Job drawing, mm, ordinate dimensions from the low corner. One solid piece. A direction names the side the tool comes from. Coordinates: 2 decimals unless noted, no trailing zeros. Order: outer loops, then holes, each group sorted by start corner. A loop starts at its lowest first (then second) coordinate and runs counter-clockwise, first axis right, second up. Notation, with made-up numbers: (-16, 53) - (28, 53) arc R19 ccw to (28, 67) - close; hole circle Ø2 at (-9.5, 74.5). An arc over 180 degrees is marked (long way). Use a Markdown table: item, result. Add a question column.
1) Tool access for the marked faces 1 and 2: list every direction of +Z, -Z, +X, -X, +Y, -Y with a clear straight run to the whole face (end or side of a thin tool).
2) Two-plate mould, pull along X, no slides. Class the marked faces 3, 4 and 5: +X half, -X half, draft (parallel to the pull), parting line (faces both ways), or undercut.
3) Saw through at D-D on y = 45. List the corners of the cut face in (x, z).
4) Saw through at A-A on y = 27.5. List the corners of the cut face in (x, z).
5) Wall check: L1, parallel to X at y = 27, z = 7 (1 decimal); L2, parallel to Y at x = 28, z = 7 (1 decimal); L3, parallel to X at y = 46, z = 4.5 (1 decimal). Give the ranges that are in metal, low to high. Write a range as [from, to].
6) Saw through at B-B on x = 27.5. List the corners of the cut face in (y, z).
7) Saw through at C-C on z = 5.75. List the corners of the cut face in (x, y).
8) Drop flat-ended pins along their axis: P1, Ø3, axis at y = 38, z = 4.5, coming from the +X side; P2, Ø4, axis at x = 13.52, y = 10.84, coming from the +Z side; P3, Ø4, axis at x = 36.5, z = 6.5, coming from the +Y side; P4, Ø4, axis at x = 12.5, z = 2, coming from the -Y side. Give the stop position or say it passes through.
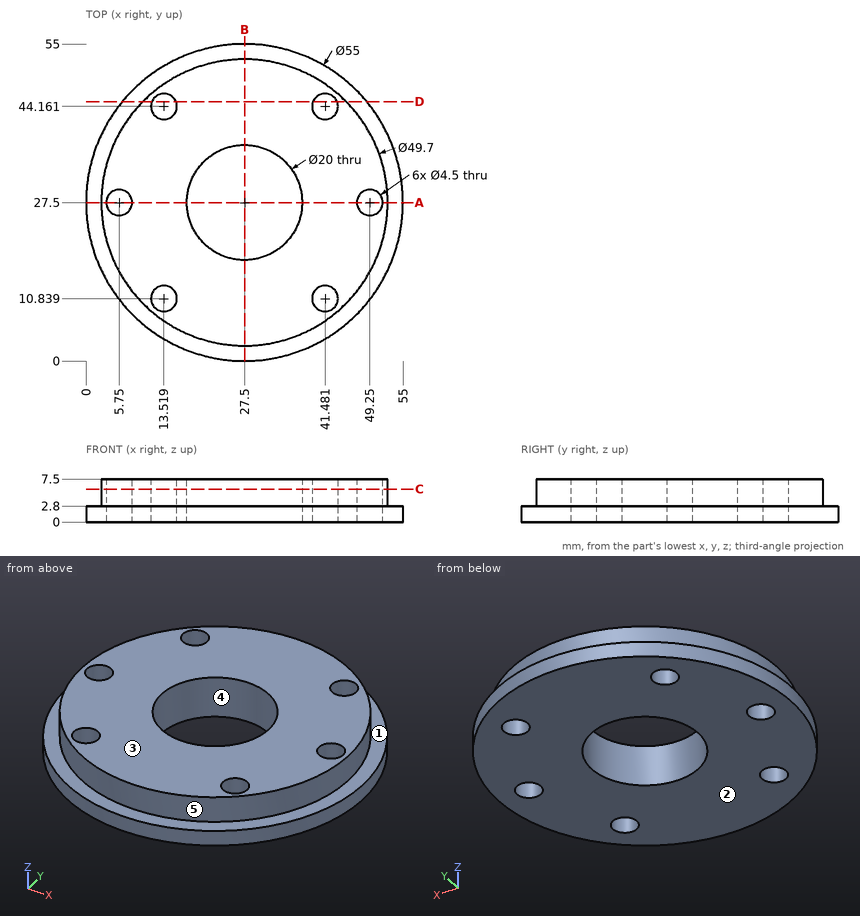
Results are:
| question | item | result |
|---|---|---|
| 1 | face 1 | +Z |
| 1 | face 2 | -Z, +X, -X, +Y, -Y |
| 2 | face 3 | draft |
| 2 | face 4 | undercut |
| 2 | face 5 | parting line |
| 3 | outline | (6.29, 0) - (11.43, 0) - (11.43, 7.5) - (9.86, 7.5) - (9.86, 2.8) - (6.29, 2.8) - close; (15.61, 0) - (39.39, 0) - (39.39, 7.5) - (15.61, 7.5) - close; (43.57, 0) - (48.71, 0) - (48.71, 2.8) - (45.14, 2.8) - (45.14, 7.5) - (43.57, 7.5) - close |
| 4 | outline | (0, 0) - (3.5, 0) - (3.5, 7.5) - (2.65, 7.5) - (2.65, 2.8) - (0, 2.8) - close; (8, 0) - (17.5, 0) - (17.5, 7.5) - (8, 7.5) - close; (37.5, 0) - (47, 0) - (47, 7.5) - (37.5, 7.5) - close; (51.5, 0) - (55, 0) - (55, 2.8) - (52.35, 2.8) - (52.35, 7.5) - (51.5, 7.5) - close |
| 5 | L1 | [2.7, 3.6], [7.9, 17.5], [37.5, 47.1], [51.4, 52.3] |
| 5 | L2 | [2.7, 17.5], [37.5, 52.3] |
| 5 | L3 | [10.9, 12.2], [14.8, 40.2], [42.8, 44.1] |
| 6 | outline | (0, 0) - (17.5, 0) - (17.5, 7.5) - (2.65, 7.5) - (2.65, 2.8) - (0, 2.8) - close; (37.5, 0) - (55, 0) - (55, 2.8) - (52.35, 2.8) - (52.35, 7.5) - (37.5, 7.5) - close |
| 7 | outline | circle Ø49.7 at (27.5, 27.5); hole circle Ø4.5 at (5.75, 27.5); hole circle Ø4.5 at (13.52, 10.84); hole circle Ø4.5 at (13.52, 44.16); hole circle Ø20 at (27.5, 27.5); hole circle Ø4.5 at (41.48, 10.84); hole circle Ø4.5 at (41.48, 44.16); hole circle Ø4.5 at (49.25, 27.5) |
| 8 | P1 | x = 50.66 |
| 8 | P2 | through |
| 8 | P3 | y = 51.34 |
| 8 | P4 | y = 3.27 |
